Part model, mm, in its own coordinate system. A direction names the side the tool comes from. Coordinates: 2 decimals unless noted, no trailing zeros. Loops run counter-clockwise (first coordinate to the right, second up) from the corner with the lowest first, then second, coordinate; pieces in that order, holes last. Notation, with made-up numbers: M 30.25,-9 L 89.25,-9 A29 ccw 89.25,16 Z; hole C 47.5,88 d2. An arc over 180 degrees is marked long. Answer as a JSON object with one key per item and string values. Group by question number.
1. 3-axis set-ups, long thin cutter, end or side, ignore diameter. For faces 1 (the face through (31.5, 11, 15)), 2 (the face through (-31.5, 11, 15)), 3 (the face through (40.53, -0.06, 1.42)): which of +Z, -Z, +X, -X, +Y, -Y reach the whole face in a straight line?
2. Mould opens along Y. For faces 4 (the face through (49, 0, 3.5)), 5 (the face through (46.12, 0.08, 0.51)) say: released by +Y, released by -Y, zero draft, split by the parting line, or undercut.
3. Drill centre lines: L1, parallel to Y at x = -29.2, z = 14.7; L2, parallel to X at y = -11, z = 14.5; L3, parallel to Y at x = -44.37, z = 2.4. Where is each one in solid material? Low to high.
4. Saw through at A-A on y = 11.7. Write the cut outline in (x, z).
5. Saw through at C-C on x = -20. Write the cut outline in (y, z), then the cut area to 3 significant figures.
6. Saw through at B-B on z = 9.5. Write the cut outline in (x, y).
7. Drop flat-ended pins along their axis: pin 1 Ø3 at (x, y) = (44.37, 0) entering from +Z; pin 2 Ø3.5 at (y, z) = (11, 14.5) entering from +X; pin 3 Ø8 at (x, y) = (-44.37, 0) entering from -Z; pin 4 Ø5 at (x, z) = (40, 7) entering from -Y. Give the stop position or say it passes through.
from build123d import *

# Parameters (mm, degrees)
SKETCH_W                      = 103
SKETCH_H                      = 9
PAD_DEPTH                     = 17
POCKET_DEPTH                  = 5.5
POCKET001_DEPTH               = 4.5
SKETCH003_W                   = 63
SKETCH003_H                   = 4.5
PAD001_DEPTH                  = 17
SKETCH005_R                   = 3
POCKET002_DEPTH               = 2.5
POCKET002_DEPTH_BACK          = 5
SKETCH006_R                   = 1.75
POCKET003_DEPTH               = 5
SKETCH007_R                   = 2
POCKET004_DEPTH               = 28
SKETCH007_MIRRORED002_2_R     = 2
POCKET004_MIRRORED002_2_DEPTH = 28
POCKET005_DEPTH               = 7
CHAMFER_SIZE                  = 1


with BuildPart() as part:
    # Sketch → Pad (new body)
    with BuildSketch(Plane.XY):
        Rectangle(SKETCH_W, SKETCH_H)
    extrude(amount=PAD_DEPTH)

    # Sketch001 → Pocket (cut, symmetric)
    with BuildSketch(Plane.XZ):
        Polygon((-39.5, 0), (-27, 12.5), (27, 12.5), (39.5, 0), align=None)
    extrude(amount=POCKET_DEPTH, both=True, mode=Mode.SUBTRACT)

    # Sketch002 → Pocket001 (cut, symmetric)
    with BuildSketch(Plane.XZ):
        Polygon((-51.88, 3.5), (-45, 3.5), (-31, 17.5), (-51.88, 17.5), align=None)
    pocket001 = extrude(amount=POCKET001_DEPTH, both=True, mode=Mode.SUBTRACT)

    # Mirrored: Pocket001 across Sketch002 V_Axis
    add(pocket001.mirror(Plane(origin=(0, 0, 0), x_dir=(0, -1, 0), z_dir=(1, 0, 0))), mode=Mode.SUBTRACT)

    # Sketch003 → Pad001 (join, symmetric)
    with BuildSketch(Plane.XZ):
        with Locations((0, 14.75)):
            Rectangle(SKETCH003_W, SKETCH003_H)
    extrude(amount=PAD001_DEPTH, both=True)

    # Sketch005 (on DatumPlane) → Pocket002 (cut, two sides)
    with BuildSketch(Plane.XY.offset(3.5)) as pocket002_sk:
        with Locations((-44.37, 0)):
            Circle(SKETCH005_R)
    pocket002 = extrude(amount=-POCKET002_DEPTH, mode=Mode.SUBTRACT) + extrude(pocket002_sk.sketch, amount=POCKET002_DEPTH_BACK, mode=Mode.SUBTRACT)

    # Sketch006 (on DatumPlane) → Pocket003 (cut)
    with BuildSketch(Plane.XY.offset(3.5)):
        with Locations((-44.37, 0)):
            Circle(SKETCH006_R)
    pocket003 = extrude(amount=-POCKET003_DEPTH, mode=Mode.SUBTRACT)

    # Mirrored001: Pocket003, Pocket002 across Sketch006 V_Axis
    add(pocket003.mirror(Plane(origin=(0, 0, 3.5), x_dir=(0, 0, 1), z_dir=(1, 0, 0))), mode=Mode.SUBTRACT)
    add(pocket002.mirror(Plane(origin=(0, 0, 3.5), x_dir=(0, 0, 1), z_dir=(1, 0, 0))), mode=Mode.SUBTRACT)

    # Sketch007 → Pocket004 (cut)
    with BuildSketch(Plane.XY):
        with Locations((-29.2, 11.7)):
            Circle(SKETCH007_R)
    pocket004 = extrude(amount=POCKET004_DEPTH, mode=Mode.SUBTRACT)

    # Sketch007 Mirrored002 2 → Pocket004 Mirrored002 2 (cut)
    with BuildSketch(Plane(origin=(0, 0, 0), x_dir=(-1, 0, 0), z_dir=(0, 0, -1))):
        with Locations((-29.2, 11.7)):
            Circle(SKETCH007_MIRRORED002_2_R)
    pocket004_mirrored002_2 = extrude(amount=-POCKET004_MIRRORED002_2_DEPTH, mode=Mode.SUBTRACT)

    # Mirrored003: Pocket004, Pocket004 Mirrored002 2 across XZ
    add(pocket004.mirror(Plane.XZ), mode=Mode.SUBTRACT)
    add(pocket004_mirrored002_2.mirror(Plane.XZ), mode=Mode.SUBTRACT)

    # Sketch008 → Pocket005 (cut, symmetric)
    with BuildSketch(Plane.XZ):
        Polygon((-41.778629, 0), (-39.243446, 2.885116), (-33.286407, 6.06738), (-33.286407, 0), align=None)
    pocket005 = extrude(amount=POCKET005_DEPTH, both=True, mode=Mode.SUBTRACT)

    # Mirrored004: Pocket005 across Sketch008 V_Axis
    add(pocket005.mirror(Plane(origin=(0, 0, 0), x_dir=(0, -1, 0), z_dir=(1, 0, 0))), mode=Mode.SUBTRACT)

    # Chamfer
    chamfer_edges = [part.edges().sort_by_distance(p)[0] for p in [
        (0, -17, 17),
        (0, 17, 17),
    ]]
    chamfer(chamfer_edges, length=CHAMFER_SIZE)


solid = part.part
Outcome:
{
 "1": {"face 1": "+Z, -Z, +X, +Y", "face 2": "+Z, -Z, -X, +Y", "face 3": "-Z, +Y, -Y"},
 "2": {"face 4": "zero draft", "face 5": "undercut"},
 "3": {"L1": "y = -17 to -13.7, -9.7 to 9.7, 13.7 to 17", "L2": "x = -31.5 to -31.07, -27.33 to 27.33, 31.07 to 31.5", "L3": "y = -4.5 to -3, 3 to 4.5"},
 "4": {"outline": "M -31.5,12.5 L -31.2,12.5 L -31.2,17 L -31.5,17 Z; M -27.2,12.5 L 27.2,12.5 L 27.2,17 L -27.2,17 Z; M 31.2,12.5 L 31.5,12.5 L 31.5,17 L 31.2,17 Z"},
 "5": {"outline": "M -17,12.5 L 17,12.5 L 17,16 L 16,17 L -16,17 L -17,16 Z", "area": "152 mm²"},
 "6": {"outline": "M -39,-4.5 L -30,-4.5 L -30,4.5 L -39,4.5 Z; M 30,-4.5 L 39,-4.5 L 39,4.5 L 30,4.5 Z"},
 "7": {"pin 1": "passes through", "pin 2": "stops at x = 31.5", "pin 3": "stops at z = 0", "pin 4": "stops at y = -4.5"}
}
